Verification items for the finished model (mm, model axes). A direction names the side the tool comes from. Give positions to 0.01 mm unless a question says otherwise; leave off trailing zeros. Write each loop counter-clockwise with the first axis right and the second up, starting at its lowest first coordinate (ties: lowest second). Pieces come first, ordered by that corner, then holes.
from build123d import *

# Parameters (mm, degrees)
F1_DEPTH      = 50
F3_DEPTH      = 20.6839429735
F3_DEPTH_BACK = 20.6839429735
F4_T          = -2
F6_DEPTH      = 25


with BuildPart() as f1:
    # F0 (on Front) → F1 (new body)
    with BuildSketch(Plane.XZ):
        Polygon((-20.175, 147.3), (-18, 0), (0, 0), (0, 147.3), align=None)
        Polygon((0, 147.3), (0, 0), (18, 0), (20.175, 147.3), align=None)
        Polygon((0, 181.7), (0, 147.3), (20.175, 147.3), (20.6829429735, 181.7), align=None)
        Polygon((-20.6829429735, 181.7), (-20.175, 147.3), (0, 147.3), (0, 181.7), align=None)
    extrude(amount=F1_DEPTH)

    # F2 (on Right) → F3 (cut, two sides)
    with BuildSketch(Plane.YZ) as f3_sk:
        Polygon((-45, 181.7), (-50, 181.7), (-50, 0), (-35, 0), align=None)
    extrude(amount=-F3_DEPTH, mode=Mode.SUBTRACT)
    extrude(f3_sk.sketch, amount=F3_DEPTH_BACK, mode=Mode.SUBTRACT)

    # F4
    f4_openings = [f1.faces().sort_by_distance(p)[0] for p in [
        (0, -22.5, 181.7),
        (0, -17.5, 0),
    ]]
    offset(amount=F4_T, openings=f4_openings)

    # F5 (on face) → F6 (cut)
    with BuildSketch(Plane(origin=(0, -34.8943073645, -1.9204351879), x_dir=(1, 0, 0), z_dir=(0, -0.9984889636, -0.0549526122))):
        Polygon((12.6829429735, 183.8983122333), (-12.6829429735, 183.8983122333), (-10, 1.9233414268), (10, 1.9233414268), align=None)
        Polygon((10, 1.9233414268), (-10, 1.9233414268), (-9.9168600221, -3.7157627956), (9.9168600221, -3.7157627956), align=None)
    extrude(amount=-F6_DEPTH, mode=Mode.SUBTRACT)


solid = f1.part
Item 1: Depth check by flat-ended pin: pin 1 (1 mm diameter, centred on y = -38.5, z = 152.5, fed in from +X); pin 2 (1 mm diameter, centred on y = -7, z = 68.5, fed in from -X); pin 3 (2 mm diameter, centred on y = -33.5, z = 161, fed in from +X). Enter the tip coordinate at first touch or a pass-through.
Answer key:
pin 1: stops at x = 20.26
pin 2: stops at x = -19.02
pin 3: stops at x = 20.39
Item 2: Sectioned sample at D-D on y = -38. Record the cut outline in (x, z) (3 decimals), then the cut area to 3 significant figures.
Answer key:
outline: (-20.683, 181.7) - (-18.805, 54.51) - (-10.805, 54.51) - (-11.341, 90.905) - (-17.342, 90.905) - (-18.683, 181.7) - close; (10.805, 54.51) - (18.805, 54.51) - (20.683, 181.7) - (18.683, 181.7) - (17.342, 90.905) - (11.341, 90.905) - close
area: 946 mm2
Item 3: Scan lines: line 1 along Y through (x, z) = (1.5, 35.5); line 2 along X through (y, z) = (-26, 162); line 3 along X through (y, z) = (-26.5, 148). Record each from-to range of solid material in increasing order.
Answer key:
line 1: y = -2 to 0
line 2: x = -20.39 to -18.39, 18.39 to 20.39
line 3: x = -20.19 to -18.19, 18.19 to 20.19
Item 4: Release check for a two-part mould opening along Y. For faces 1 (the face through (0, -2, 92)), 2 (the face through (15.27, -39.93, 89.58)), 3 (the face through (0, 0, 92)) record: released by +Y, released by -Y, zero draft, split by the parting line, or undercut.
Answer key:
face 1: undercut
face 2: released by -Y
face 3: released by +Y
Item 5: Sectioned sample at B-B on z = 98. Record the cut outline in (x, y).
Answer key:
outline: (-19.45, -40.39) - (-11.45, -40.39) - (-11.45, -38.39) - (-17.45, -38.39) - (-17.45, -2) - (17.45, -2) - (17.45, -38.39) - (11.45, -38.39) - (11.45, -40.39) - (19.45, -40.39) - (19.45, 0) - (-19.45, 0) - close
Item 6: Set-up check for faces 4 (the face through (0, -1, 181.7)), 5 (the face through (14.28, -37.927, 89.578)): record each of +Z, -Z, +X, -X, +Y, -Y from which the full face is reachable in a straight line by a thin tool's end or side.
Answer key:
face 4: +Z, +X, -X, +Y, -Y
face 5: +Z
Item 7: Sectioned sample at C-C on x = 4.5. Record the cut outline in (y, z).
Answer key:
outline: (-2, 0) - (0, 0) - (0, 181.7) - (-2, 181.7) - close
Item 8: Sectioned sample at A-A on y = -30. Record the cut outline in (x, z), then the cut area to 3 significant figures.
Answer key:
outline: (-20.68, 181.7) - (-18, 0) - (-16, 0) - (-18.68, 181.7) - close; (16, 0) - (18, 0) - (20.68, 181.7) - (18.68, 181.7) - close
area: 727 mm2
